Input: part model. Units: mm. Frame: model coordinates. Face numbers are marked on the shaded views. A direction names the side the tool comes from. Coordinates: 2 decimals unless noted, no trailing zeros. Order: outer loops, then holes, each group sorted by start corner. A loop starts at its lowest first (then second) coordinate and runs counter-clockwise, first axis right, second up. Notation, with made-up numbers: M -39.5,-34.75 L -1.5,-34.75 A17 ccw -1.5,-27.75 Z; hole C -24,82.5 d5. An arc over 180 degrees is marked long. One line per item, written item: value.
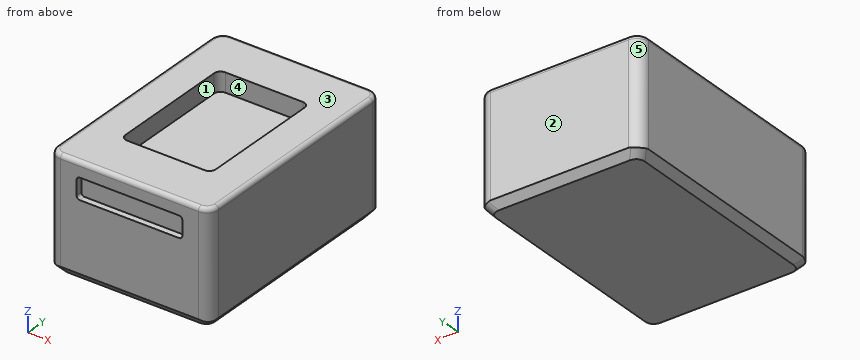
```python
from build123d import *

# Parameters (mm, degrees)
SKETCH2_W           = 76.2
SKETCH2_H           = 109.22
BOSS_EXTRUDE1_DEPTH = 53.34
CHAMFER1_SIZE       = 3
CHAMFER1_SIZE2      = 3.575260778
CHAMFER2_SIZE       = 3
CHAMFER2_SIZE2      = 3.575260778
FILLET2_R           = 5.5
FILLET3_R           = 5.5
FILLET4_R           = 2
CUT_EXTRUDE1_DEPTH  = 9
CUT_EXTRUDE2_DEPTH  = 3


with BuildPart() as part:
    # Sketch2 → Boss-Extrude1 (new body)
    with BuildSketch(Plane.XY):
        with Locations((38.1, 54.61)):
            Rectangle(SKETCH2_W, SKETCH2_H)
    extrude(amount=BOSS_EXTRUDE1_DEPTH)

    # Chamfer1
    chamfer1_edges = [part.edges().sort_by_distance(p)[0] for p in [
        (38.1, 109.22, 0),
    ]]
    chamfer1_side = [part.faces().sort_by_distance(p)[0] for p in [
        (38.1, 54.61, 0),
    ]]
    chamfer(chamfer1_edges, length=CHAMFER1_SIZE, length2=CHAMFER1_SIZE2, reference=chamfer1_side[0])

    # Chamfer2
    chamfer2_edges = [part.edges().sort_by_distance(p)[0] for p in [
        (0, 53.11, 0),
        (38.1, 0, 0),
        (76.2, 53.11, 0),
    ]]
    chamfer2_side = [part.faces().sort_by_distance(p)[0] for p in [
        (38.1, 53.11, 0),
    ]]
    chamfer(chamfer2_edges, length=CHAMFER2_SIZE, length2=CHAMFER2_SIZE2, reference=chamfer2_side[0])

    # Fillet2
    fillet2_edges = [part.edges().sort_by_distance(p)[0] for p in [
        (74.7, 107.72, 1.787630389),
        (1.5, 107.72, 1.787630389),
        (74.7, 1.5, 1.787630389),
        (1.5, 1.5, 1.787630389),
    ]]
    fillet(fillet2_edges, radius=FILLET2_R)

    # Fillet3
    fillet3_edges = [part.edges().sort_by_distance(p)[0] for p in [
        (76.2, 0, 29.139633853),
        (0, 0, 29.139633853),
        (0, 109.22, 29.139633853),
        (76.2, 109.22, 29.139633853),
    ]]
    fillet(fillet3_edges, radius=FILLET3_R - 0.0001)  # a hair under: the kernel refuses the full size

    # Fillet4
    fillet4_edges = [part.edges().sort_by_distance(p)[0] for p in [
        (76.2, 54.61, 53.34),
        (38.1, 0, 53.34),
        (0, 54.61, 53.34),
        (38.1, 109.22, 53.34),
        (74.589116586, 107.609116586, 53.34),
        (1.610883414, 107.609116586, 53.34),
        (1.610883414, 1.610883414, 53.34),
        (74.589116586, 1.610883414, 53.34),
    ]]
    fillet(fillet4_edges, radius=FILLET4_R)

    # Sketch4 → Cut-Extrude1 (cut)
    with BuildSketch(Plane.XY.offset(53.34)):
        with BuildLine():
            Line((19.741636299, 85.947770103), (56.458363701, 85.947770103))
            ThreePointArc((56.458363701, 85.947770103), (58.579684045, 85.069090446), (59.458363701, 82.947770103))
            Line((59.458363701, 82.947770103), (59.458363701, 26.272229897))
            ThreePointArc((59.458363701, 26.272229897), (58.579684045, 24.150909554), (56.458363701, 23.272229897))
            Line((56.458363701, 23.272229897), (19.741636299, 23.272229897))
            ThreePointArc((19.741636299, 23.272229897), (17.620315955, 24.150909554), (16.741636299, 26.272229897))
            Line((16.741636299, 26.272229897), (16.741636299, 82.947770103))
            ThreePointArc((16.741636299, 82.947770103), (17.620315955, 85.069090446), (19.741636299, 85.947770103))
        make_face()
    extrude(amount=-CUT_EXTRUDE1_DEPTH, mode=Mode.SUBTRACT)

    # Sketch5 → Cut-Extrude2 (cut)
    with BuildSketch(Plane.XZ):
        with BuildLine():
            Line((14.6, 36.34), (61.6, 36.34))
            ThreePointArc((61.6, 36.34), (62.660660172, 36.779339828), (63.1, 37.84))
            Line((63.1, 37.84), (63.1, 44.84))
            ThreePointArc((63.1, 44.84), (62.660660172, 45.900660172), (61.6, 46.34))
            Line((61.6, 46.34), (14.6, 46.34))
            ThreePointArc((14.6, 46.34), (13.539339828, 45.900660172), (13.1, 44.84))
            Line((13.1, 44.84), (13.1, 37.84))
            ThreePointArc((13.1, 37.84), (13.539339828, 36.779339828), (14.6, 36.34))
        make_face()
    extrude(amount=-CUT_EXTRUDE2_DEPTH, mode=Mode.SUBTRACT)


solid = part.part
```
(1) Cut plane C-C on y = 25. Output: boundary loops of the cut face in (x, z), plus the area to 3 significant figures.
Data:
outline: M 0,3.58 L 3,0 L 73.2,0 L 76.2,3.58 L 76.2,51.34 A2 ccw 74.2,53.34 L 59.18,53.34 L 59.18,44.34 L 17.02,44.34 L 17.02,53.34 L 2,53.34 A2 ccw 0,51.34 Z
area: 3,670 mm2
(2) Access query for the marked faces 4 and 5. Directions: +Z, -Z, +X, -X, +Y, -Y. A direction counts if a zero-diameter tool reaches every point of the face in a straight line with its end or side. Return the directions, or none.
Data:
face 4: +Z
face 5: +Z, -Z, -X, +Y
(3) Cut plane A-A on y = 56.5. Output: boundary loops of the cut face in (x, z), plus the area to 3 significant figures.
Data:
outline: M 0,3.58 L 3,0 L 73.2,0 L 76.2,3.58 L 76.2,51.34 A2 ccw 74.2,53.34 L 59.46,53.34 L 59.46,44.34 L 16.74,44.34 L 16.74,53.34 L 2,53.34 A2 ccw 0,51.34 Z
area: 3,670 mm2
(4) Draft query along Y for the marked faces 1, 2 and 3. Return one class per face: released by +Y, released by -Y, zero draft, split by the parting line, or undercut.
Data:
face 1: undercut
face 2: released by +Y
face 3: zero draft
(5) First-contact query: pin 1 (21.5 mm diameter, centred on x = 32, y = 65, fed in from +Z); pin 2 (1.5 mm diameter, centred on y = 1, z = 42.5, fed in from +X); pin 3 (3.5 mm diameter, centred on y = 1.5, z = 42.5, fed in from -X). Flat tips, straight axial feed; report the tip coordinate or a pass-through.
Data:
pin 1: stops at z = 44.34
pin 2: stops at x = 74.72
pin 3: stops at x = 0.48
(6) Cut plane B-B on x = 34.5. Output: boundary loops of the cut face in (y, z).
Data:
outline: M 0,3.58 L 3,0 L 106.22,0 L 109.22,3.58 L 109.22,51.34 A2 ccw 107.22,53.34 L 85.95,53.34 L 85.95,44.34 L 23.27,44.34 L 23.27,53.34 L 2,53.34 A2 ccw 0,51.34 L 0,46.34 L 3,46.34 L 3,36.34 L 0,36.34 Z
(7) Ray query, line 1 (Y direction, x = 56, z = 47); line 2 (X direction, y = 43, z = 50); line 3 (Y direction, x = 34, z = 41.5). Return the intervals inside material, ascending. Write a range as from..to.
Data:
line 1: y = 0..23.27, 85.95..109.22
line 2: x = 0..16.74, 59.46..76.2
line 3: y = 3..109.22
